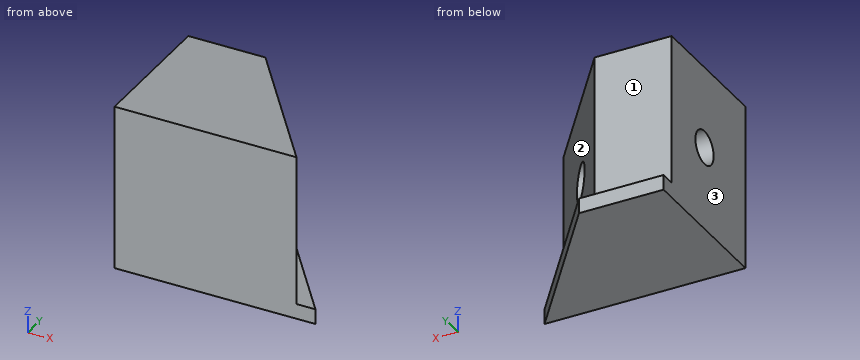
```python
from build123d import *

# Parameters (mm, degrees)
F1_DEPTH = 6.35
F3_DEPTH = 63.5
F4_R     = 7.097159
F5_DEPTH = 159.004


with BuildPart() as f1:
    # F0 (on Top) → F1 (new body)
    with BuildSketch(Plane.XY):
        Polygon((-6.691513, 31.987395), (-42.290725, 31.987395), (-42.290725, -31.987395), (42.290725, -31.987395), align=None)
    extrude(amount=F1_DEPTH)

    # F2 (on face) → F3 (join)
    with BuildSketch(Plane.XY.offset(6.35)):
        Polygon((-9.82716, 25.637395), (-42.290725, 25.637395), (-42.290725, -31.987395), (34.293207, -31.987395), align=None)
    extrude(amount=F3_DEPTH)

    # F4 (on face) → F5 (cut)
    with BuildSketch(Plane(origin=(-42.290725, 0, 0), x_dir=(0, -1, 0), z_dir=(-1, 0, 0))):
        with Locations((0, 35.157394)):
            Circle(F4_R)
    extrude(amount=-F5_DEPTH, mode=Mode.SUBTRACT)


solid = f1.part
```
Work out the finished part from the listing and answer in its coordinate system (mm). Face numbers are marked on the shaded views. A direction names the side the tool comes from. Round coordinates to 2 decimals unless told otherwise and drop trailing zeros. Order: outer loops, then holes, each group sorted by start corner. A loop starts at its lowest first (then second) coordinate and runs counter-clockwise, first axis right, second up.
Q1. A cutting plane is placed at D-D, the plane x = -29.5. Determine the outline of the cut face in (y, z), then the cut area to 3 significant figures.
Solution:
outline: (-31.99, 0) - (31.99, 0) - (31.99, 6.35) - (25.64, 6.35) - (25.64, 69.85) - (-31.99, 69.85) - close; hole circle Ø14.19 at (0, 35.16)
area: 3,910 mm2
Q2. A cutting plane is placed at A-A, the plane z = 39. Determine the outline of the cut face in (x, y).
Solution:
outline: (-42.29, -31.99) - (34.29, -31.99) - (14.37, -5.97) - (-42.29, -5.97) - close; (-42.29, 5.97) - (5.23, 5.97) - (-9.83, 25.64) - (-42.29, 25.64) - close
Q3. Find the intervals of material crossed by line 1 along Z through (x, y) = (-24, 0); line 2 along Y through (x, z) = (-25, 35); line 3 along Y through (x, z) = (-15.5, 64.5), in increasing order.
Solution:
line 1: z = 0 to 28.06, 42.25 to 69.85
line 2: y = -31.99 to -7.1, 7.1 to 25.64
line 3: y = -31.99 to 25.64
Q4. A cutting plane is placed at C-C, the plane x = 4.5. Determine the outline of the cut face in (y, z).
Solution:
outline: (-31.99, 0) - (17.37, 0) - (17.37, 6.35) - (6.92, 6.35) - (6.92, 33.6) arc R7.1 cw (long way) to (6.92, 36.71) - (6.92, 69.85) - (-31.99, 69.85) - close
Q5. Given pin 1 Ø3 at (x, y) = (7.5, 7) entering from +Z; pin 2 Ø3 at (y, z) = (22, 14) entering from +X; pin 3 Ø4 at (y, z) = (4, 22.5) entering from +X, each flat-ended and moving along its own axis, determine where each tip first touches the part or whether it passes through.
Solution:
pin 1: stops at z = 6.35
pin 2: stops at x = -5.89
pin 3: stops at x = 8.27
Q6. A cutting plane is placed at B-B, the plane y = 0. Determine the outline of the cut face in (x, z).
Solution:
outline: (-42.29, 0) - (17.8, 0) - (17.8, 6.35) - (9.8, 6.35) - (9.8, 28.06) - (-42.29, 28.06) - close; (-42.29, 42.25) - (9.8, 42.25) - (9.8, 69.85) - (-42.29, 69.85) - close
Q7. A tool of negligible diameter and unlimited length cuts with its end or side. For the marked faces 1, 2 and 3, from which of +Z, -Z, +X, -X, +Y, -Y can it reach the whole face along a straight path? Write none if from no direction.
Solution:
face 1: +Z, +X, -X, +Y
face 2: +Z, +X, +Y
face 3: +Z, -Z, -X, +Y, -Y
